Verification items for the finished model (mm, model axes). Coordinates: 2 decimals unless noted, no trailing zeros. Write each question's results on one line, items separated by ' | '. Start each with the question number.
(1) Cross-section at A-A on y = 2.25. Give the number of separate pieces and of enclosed holes in the cut face, and give its area (3 significant figures).
(2) Thickness scan on probe 1 along X at (y, z) = (2.75, -117); probe 2 along X at (y, z) = (0.5, -16); probe 3 along X at (y, z) = (3, -41.63). Record the ranges inside material, lowest first. Write a range as [from, to].
(3) Go/stop test with a flat-tipped pin: pin 1 (2 mm diameter, centred on x = 122.7, z = -63.13, fed in from -Y) (3 decimals). Record where the tip stops, or that it passes through.
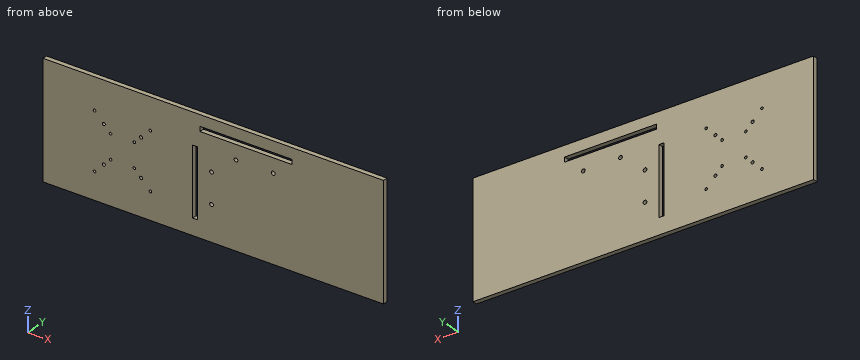
```python
from build123d import *

# Parameters (mm, degrees)
SKETCH1_W           = 457.2
SKETCH1_H           = 152.4
SKETCH1_R           = 1.75
SKETCH1_R_2         = 2.5
SKETCH1_R_3         = 2
SKETCH1_W_2         = 123.32
SKETCH1_H_2         = 6.35
SKETCH1_W_3         = 6.35
SKETCH1_H_3         = 90
BOSS_EXTRUDE1_DEPTH = 6.35


with BuildPart() as part:
    # Sketch1 → Boss-Extrude1 (new body)
    with BuildSketch(Plane(origin=(0, 0, 0), x_dir=(1, 0, 0), z_dir=(0, 1, 0))):
        with Locations((228.6, 76.2)):
            Rectangle(SKETCH1_W, SKETCH1_H)
        with Locations(Location((90.702581284, 95.13, 0), (0, 0, 270))):
            Circle(SKETCH1_R, mode=Mode.SUBTRACT)
        with Locations(Location((122.702581284, 95.13, 0), (0, 0, 270))):
            Circle(SKETCH1_R, mode=Mode.SUBTRACT)
        with Locations(Location((122.702581284, 63.13, 0), (0, 0, 270))):
            Circle(SKETCH1_R, mode=Mode.SUBTRACT)
        with Locations(Location((90.702581284, 63.13, 0), (0, 0, 270))):
            Circle(SKETCH1_R, mode=Mode.SUBTRACT)
        with Locations(Location((69.202581284, 116.63, 0), (0, 0, 270))):
            Circle(SKETCH1_R, mode=Mode.SUBTRACT)
        with Locations(Location((144.202581284, 116.63, 0), (0, 0, 270))):
            Circle(SKETCH1_R, mode=Mode.SUBTRACT)
        with Locations(Location((144.202581284, 41.63, 0), (0, 0, 270))):
            Circle(SKETCH1_R, mode=Mode.SUBTRACT)
        with Locations(Location((69.202581284, 41.63, 0), (0, 0, 270))):
            Circle(SKETCH1_R, mode=Mode.SUBTRACT)
        with Locations(Location((226.25, 65.86, 0), (0, 0, 270))):
            Circle(SKETCH1_R_2, mode=Mode.SUBTRACT)
        with Locations(Location((226.25, 105.86, 0), (0, 0, 270))):
            Circle(SKETCH1_R_2, mode=Mode.SUBTRACT)
        with Locations(Location((259.17, 39.91, 0), (0, 0, 270))):
            Circle(SKETCH1_R_2, mode=Mode.SUBTRACT)
        with Locations(Location((309.17, 39.91, 0), (0, 0, 270))):
            Circle(SKETCH1_R_2, mode=Mode.SUBTRACT)
        with Locations(Location((81.702581284, 104.13, 0), (0, 0, 270))):
            Circle(SKETCH1_R_3, mode=Mode.SUBTRACT)
        with Locations(Location((131.702581284, 104.13, 0), (0, 0, 270))):
            Circle(SKETCH1_R_3, mode=Mode.SUBTRACT)
        with Locations(Location((131.702581284, 54.13, 0), (0, 0, 270))):
            Circle(SKETCH1_R_3, mode=Mode.SUBTRACT)
        with Locations(Location((81.702581284, 54.13, 0), (0, 0, 270))):
            Circle(SKETCH1_R_3, mode=Mode.SUBTRACT)
        with Locations((272.51, 17.685)):
            Rectangle(SKETCH1_W_2, SKETCH1_H_2, mode=Mode.SUBTRACT)
        with Locations((204.025, 85.86)):
            Rectangle(SKETCH1_W_3, SKETCH1_H_3, mode=Mode.SUBTRACT)
    extrude(amount=BOSS_EXTRUDE1_DEPTH)


solid = part.part
```
Results are:
1) separate pieces: 1 | enclosed holes: 18 | area: 68,100 mm2
2) probe 1: x = [0, 67.49], [70.91, 142.49], [145.91, 200.85], [207.2, 457.2] | probe 2: x = [0, 210.85], [334.17, 457.2] | probe 3: x = [0, 67.45], [70.95, 142.45], [145.95, 200.85], [207.2, 257.36], [260.98, 307.36], [310.98, 457.2]
3) pin 1: passes through
